from build123d import *

# Parameters (mm, degrees)
SCHIZZO1_R                   = 3.375
ESTRUSIONE_ESTRUSIONE1_DEPTH = 1.35
SCHIZZO2_R                   = 3.375
ESTRUSIONE_ESTRUSIONE2_DEPTH = 2
SCHIZZO3_R                   = 2.25
TAGLIO_ESTRUSIONE1_DEPTH     = 2
SCHIZZO4_R                   = 1.2
TAGLIO_ESTRUSIONE2_DEPTH     = 21.102984853
SCHIZZO5_R                   = 0.5
TAGLIO_ESTRUSIONE3_DEPTH     = 21.281826841


with BuildPart() as part:
    # Schizzo1 → Estrusione-Estrusione1 (new body)
    with BuildSketch(Plane(origin=(0, 0, 0), x_dir=(1, 0, 0), z_dir=(0, 1, 0))):
        Circle(SCHIZZO1_R)
        with BuildLine():
            Line((-1.846618531, 2.825), (-14.5, 1.5))
            ThreePointArc((-14.5, 1.5), (-16, 0), (-14.5, -1.5))
            Line((-14.5, -1.5), (-1.846618531, -2.825))
            Line((-1.846618531, -2.825), (-1.846618531, 2.825))
        make_face()
        with BuildLine():
            Line((1.85, 3.45), (1.85, -3.45))
            Line((1.85, -3.45), (16.7, -1.5))
            ThreePointArc((16.7, -1.5), (18.2, 0), (16.7, 1.5))
            Line((16.7, 1.5), (1.85, 3.45))
        make_face()
        with BuildLine():
            Line((-1.85, -6.45), (-1.85, 6.45))
            ThreePointArc((-1.85, 6.45), (0, 8.3), (1.85, 6.45))
            Line((1.85, 6.45), (1.85, -6.45))
            ThreePointArc((1.85, -6.45), (0, -8.3), (-1.85, -6.45))
        make_face()
    extrude(amount=ESTRUSIONE_ESTRUSIONE1_DEPTH)

    # Schizzo2 → Estrusione-Estrusione2 (add)
    with BuildSketch(Plane(origin=(0, 1.35, 0), x_dir=(1, 0, 0), z_dir=(0, 1, 0))):
        with Locations(Location((0, 0, 0), (0, 0, 270))):
            Circle(SCHIZZO2_R)
    extrude(amount=ESTRUSIONE_ESTRUSIONE2_DEPTH)

    # Schizzo3 → Taglio-Estrusione1 (cut)
    with BuildSketch(Plane(origin=(0, 3.35, 0), x_dir=(1, 0, 0), z_dir=(0, 1, 0))):
        with Locations(Location((0, 0, 0), (0, 0, 270))):
            Circle(SCHIZZO3_R)
    extrude(amount=-TAGLIO_ESTRUSIONE1_DEPTH, mode=Mode.SUBTRACT)

    # Schizzo4 → Taglio-Estrusione2 (cut, through all)
    with BuildSketch(Plane(origin=(0, 1.35, 0), x_dir=(1, 0, 0), z_dir=(0, 1, 0))):
        with Locations(Location((0, 0, 0), (0, 0, 270))):
            Circle(SCHIZZO4_R)
    extrude(amount=-TAGLIO_ESTRUSIONE2_DEPTH, mode=Mode.SUBTRACT)

    # Schizzo5 → Taglio-Estrusione3 (cut, through all)
    with BuildSketch(Plane.XZ):
        with Locations(Location((8.7, 0, 0), (0, 0, 270))):
            Circle(SCHIZZO5_R)
        with Locations(Location((10.7, 0, 0), (0, 0, 270))):
            Circle(SCHIZZO5_R)
        with Locations(Location((12.7, 0, 0), (0, 0, 270))):
            Circle(SCHIZZO5_R)
        with Locations(Location((14.7, 0, 0), (0, 0, 270))):
            Circle(SCHIZZO5_R)
        with Locations(Location((16.7, 0, 0), (0, 0, 270))):
            Circle(SCHIZZO5_R)
        with Locations(Location((6.7, 0, 0), (0, 0, 270))):
            Circle(SCHIZZO5_R)
        with Locations(Location((4.7, 0, 0), (0, 0, 270))):
            Circle(SCHIZZO5_R)
        with Locations(Location((0, 4.4, 0), (0, 0, 270))):
            Circle(SCHIZZO5_R)
        with Locations(Location((0, 6.4, 0), (0, 0, 270))):
            Circle(SCHIZZO5_R)
    extrude(amount=-TAGLIO_ESTRUSIONE3_DEPTH, mode=Mode.SUBTRACT)


solid = part.part
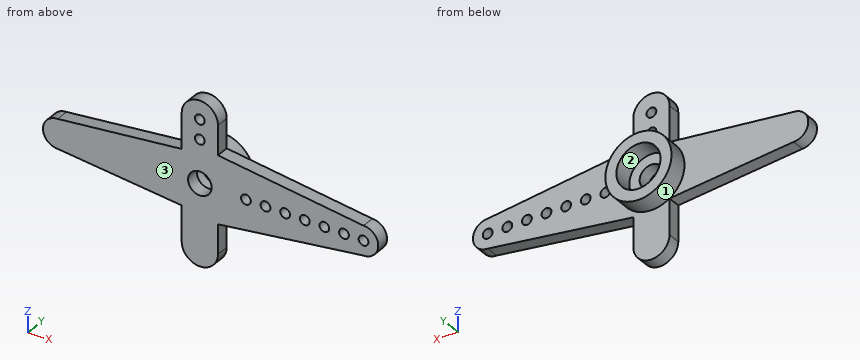
The model under review builds one solid part; all positions refer to its coordinate system, in mm. Face numbers are marked on the shaded views. Round coordinates to 2 decimals unless told otherwise and drop trailing zeros. Loops run counter-clockwise (first coordinate to the right, second up) from the corner with the lowest first, then second, coordinate; pieces in that order, holes last. Notation, with made-up numbers: (46.25, 48) -> (56.25, 48) arc R17 ccw to (56.25, 53) -> close; hole circle Ø8 at (26, 56.5). An arc over 180 degrees is marked (long way). Return JSON: item names as keys, results as strings.
(1) For pin 1 (3 mm diameter, centred on x = 4.5, z = 6, fed in from -Y); pin 2 (0.7 mm diameter, centred on y = 1, z = 5, fed in from +X); pin 3 (2 mm diameter, centred on x = -0.5, z = 0, fed in from +Y); pin 4 (0.7 mm diameter, centred on y = 1, z = 4.5, fed in from -X), all flat-tipped, find the tip position at first contact; note any pin that passes through.
Solved:
{"pin 1": "through", "pin 2": "x = 1.85", "pin 3": "y = 1.35", "pin 4": "x = -1.85"}
(2) Add section C-C on x = 8.7. Write out the cut boundary in (y, z).
Solved:
{"outline": "(0, -2.55) -> (1.35, -2.55) -> (1.35, -0.5) -> (0, -0.5) -> close; (0, 0.5) -> (1.35, 0.5) -> (1.35, 2.55) -> (0, 2.55) -> close"}
(3) For line 1 (X direction, y = 0.7, z = 6.4); line 2 (X direction, y = 0.85, z = 5); line 3 (Y direction, x = 12, z = -0.5), list the stretches that pass through material, from the lowest coordinate up.
Solved:
{"line 1": "-1.85 to -0.5, 0.5 to 1.85", "line 2": "-1.85 to 1.85", "line 3": "0 to 1.35"}
(4) Add section A-A on y = 0.6. State how many separate pieces and enclosed holes the cut face has, plus the area to 3 significant figures.
Solved:
{"separate pieces": "1", "enclosed holes": "10", "area": "182 mm2"}
(5) Add section D-D on y = 2.5. Write out the cut boundary in (x, z) (3 decimals).
Solved:
{"outline": "circle Ø6.75 at (0, 0); hole circle Ø4.5 at (0, 0)"}
(6) The part is to be moulded in two halves that separate along X. For the marked faces 1, 2 and 3, say which applies: released by +X, released by -X, zero draft, split by the parting line, or undercut.
Solved:
{"face 1": "split by the parting line", "face 2": "undercut", "face 3": "zero draft"}
(7) Add section B-B on z = 4.4. Write out the cut boundary in (x, y), plus the area to 4 significant figures.
Solved:
{"outline": "(-1.85, 0) -> (-0.5, 0) -> (-0.5, 1.35) -> (-1.85, 1.35) -> close; (0.5, 0) -> (1.85, 0) -> (1.85, 1.35) -> (0.5, 1.35) -> close", "area": "3.645 mm2"}
